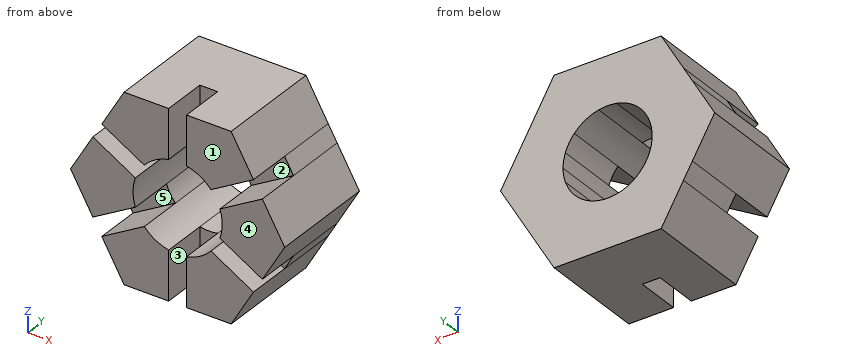
from build123d import *

# Parameters (mm, degrees)
BOSS_EXTRUDE1_DEPTH = 60
CUT_EXTRUDE1_DEPTH  = 25


with BuildPart() as part:
    # Sketch1 → Boss-Extrude1 (new body)
    with BuildSketch(Plane(origin=(0, 0, 0), x_dir=(1, 0, 0), z_dir=(0, 1, 0))):
        with BuildLine():
            Line((-47.533320997, 21.669872981), (-23.713203436, 7.917321695))
            ThreePointArc((-23.713203436, 7.917321695), (-21.650635095, 12.5), (-18.713203436, 16.577575733))
            Line((-18.713203436, 16.577575733), (-42.533320997, 30.330127019))
            Line((-42.533320997, 30.330127019), (-47.533320997, 21.669872981))
        make_face()
        with BuildLine():
            Line((-42.533320997, 30.330127019), (-18.713203436, 16.577575733))
            ThreePointArc((-18.713203436, 16.577575733), (-12.5, 21.650635095), (-5, 24.494897428))
            Line((-5, 24.494897428), (-5, 52))
            Line((-5, 52), (-30.022213998, 52))
            Line((-30.022213998, 52), (-42.533320997, 30.330127019))
        make_face()
        with BuildLine():
            Line((5, 24.494897428), (5, 52))
            Line((5, 52), (-5, 52))
            Line((-5, 52), (-5, 24.494897428))
            ThreePointArc((-5, 24.494897428), (0, 25), (5, 24.494897428))
        make_face()
        with BuildLine():
            Line((18.713203436, 16.577575733), (42.533320997, 30.330127019))
            Line((42.533320997, 30.330127019), (30.022213998, 52))
            Line((30.022213998, 52), (5, 52))
            Line((5, 52), (5, 24.494897428))
            ThreePointArc((5, 24.494897428), (12.5, 21.650635095), (18.713203436, 16.577575733))
        make_face()
        with BuildLine():
            Line((23.713203436, 7.917321695), (47.533320997, 21.669872981))
            Line((47.533320997, 21.669872981), (42.533320997, 30.330127019))
            Line((42.533320997, 30.330127019), (18.713203436, 16.577575733))
            ThreePointArc((18.713203436, 16.577575733), (21.650635095, 12.5), (23.713203436, 7.917321695))
        make_face()
        with BuildLine():
            Line((23.713203436, -7.917321695), (47.533320997, -21.669872981))
            Line((47.533320997, -21.669872981), (60.044427996, 0))
            Line((60.044427996, 0), (47.533320997, 21.669872981))
            Line((47.533320997, 21.669872981), (23.713203436, 7.917321695))
            ThreePointArc((23.713203436, 7.917321695), (24.676203982, 4.010605572), (25, 0))
            ThreePointArc((25, 0), (24.676203982, -4.010605572), (23.713203436, -7.917321695))
        make_face()
        with BuildLine():
            Line((18.713203436, -16.577575733), (42.533320997, -30.330127019))
            Line((42.533320997, -30.330127019), (47.533320997, -21.669872981))
            Line((47.533320997, -21.669872981), (23.713203436, -7.917321695))
            ThreePointArc((23.713203436, -7.917321695), (21.650635095, -12.5), (18.713203436, -16.577575733))
        make_face()
        with BuildLine():
            Line((5, -52), (30.022213998, -52))
            Line((30.022213998, -52), (42.533320997, -30.330127019))
            Line((42.533320997, -30.330127019), (18.713203436, -16.577575733))
            ThreePointArc((18.713203436, -16.577575733), (12.5, -21.650635095), (5, -24.494897428))
            Line((5, -24.494897428), (5, -52))
        make_face()
        with BuildLine():
            Line((-5, -52), (5, -52))
            Line((5, -52), (5, -24.494897428))
            ThreePointArc((5, -24.494897428), (0, -25), (-5, -24.494897428))
            Line((-5, -24.494897428), (-5, -52))
        make_face()
        with BuildLine():
            Line((-30.022213998, -52), (-5, -52))
            Line((-5, -52), (-5, -24.494897428))
            ThreePointArc((-5, -24.494897428), (-12.5, -21.650635095), (-18.713203436, -16.577575733))
            Line((-18.713203436, -16.577575733), (-42.533320997, -30.330127019))
            Line((-42.533320997, -30.330127019), (-30.022213998, -52))
        make_face()
        with BuildLine():
            Line((-47.533320997, -21.669872981), (-42.533320997, -30.330127019))
            Line((-42.533320997, -30.330127019), (-18.713203436, -16.577575733))
            ThreePointArc((-18.713203436, -16.577575733), (-21.650635095, -12.5), (-23.713203436, -7.917321695))
            Line((-23.713203436, -7.917321695), (-47.533320997, -21.669872981))
        make_face()
        with BuildLine():
            Line((-60.044427996, 0), (-47.533320997, -21.669872981))
            Line((-47.533320997, -21.669872981), (-23.713203436, -7.917321695))
            ThreePointArc((-23.713203436, -7.917321695), (-25, 0), (-23.713203436, 7.917321695))
            Line((-23.713203436, 7.917321695), (-47.533320997, 21.669872981))
            Line((-47.533320997, 21.669872981), (-60.044427996, 0))
        make_face()
    extrude(amount=BOSS_EXTRUDE1_DEPTH)

    # Sketch1_4 → Cut-Extrude1 (cut)
    with BuildSketch(Plane(origin=(0, 0, 0), x_dir=(1, 0, 0), z_dir=(0, 1, 0))):
        with BuildLine():
            Line((-47.533320997, 21.669872981), (-23.713203436, 7.917321695))
            ThreePointArc((-23.713203436, 7.917321695), (-21.650635095, 12.5), (-18.713203436, 16.577575733))
            Line((-18.713203436, 16.577575733), (-42.533320997, 30.330127019))
            Line((-42.533320997, 30.330127019), (-47.533320997, 21.669872981))
        make_face()
        with BuildLine():
            Line((-47.533320997, -21.669872981), (-42.533320997, -30.330127019))
            Line((-42.533320997, -30.330127019), (-18.713203436, -16.577575733))
            ThreePointArc((-18.713203436, -16.577575733), (-21.650635095, -12.5), (-23.713203436, -7.917321695))
            Line((-23.713203436, -7.917321695), (-47.533320997, -21.669872981))
        make_face()
        with BuildLine():
            Line((-5, -52), (5, -52))
            Line((5, -52), (5, -24.494897428))
            ThreePointArc((5, -24.494897428), (0, -25), (-5, -24.494897428))
            Line((-5, -24.494897428), (-5, -52))
        make_face()
        with BuildLine():
            Line((18.713203436, -16.577575733), (42.533320997, -30.330127019))
            Line((42.533320997, -30.330127019), (47.533320997, -21.669872981))
            Line((47.533320997, -21.669872981), (23.713203436, -7.917321695))
            ThreePointArc((23.713203436, -7.917321695), (21.650635095, -12.5), (18.713203436, -16.577575733))
        make_face()
        with BuildLine():
            Line((23.713203436, 7.917321695), (47.533320997, 21.669872981))
            Line((47.533320997, 21.669872981), (42.533320997, 30.330127019))
            Line((42.533320997, 30.330127019), (18.713203436, 16.577575733))
            ThreePointArc((18.713203436, 16.577575733), (21.650635095, 12.5), (23.713203436, 7.917321695))
        make_face()
        with BuildLine():
            Line((5, 24.494897428), (5, 52))
            Line((5, 52), (-5, 52))
            Line((-5, 52), (-5, 24.494897428))
            ThreePointArc((-5, 24.494897428), (0, 25), (5, 24.494897428))
        make_face()
    extrude(amount=CUT_EXTRUDE1_DEPTH, mode=Mode.SUBTRACT)


solid = part.part
Could you check a few things on this model? Use its own coordinates, in mm. Face numbers are marked on the shaded views. A direction names the side the tool comes from. Give positions to 0.01 mm unless a question says otherwise; leave off trailing zeros. Order: outer loops, then holes, each group sorted by start corner. A loop starts at its lowest first (then second) coordinate and runs counter-clockwise, first axis right, second up. Notation, with made-up numbers: (37.5, 87) -> (62.5, 87) arc R11 cw to (62.5, 106) -> close; hole circle Ø9 at (-34, 24.25). An arc over 180 degrees is marked (long way). Answer in a Markdown table with one row per item. Add a question column.
Item 1: For the marked faces 1, 2 and 3, which set-ups out of +Z, -Z, +X, -X, +Y, -Y let a thin tool reach every point of the face, with its end or its side?
Item 2: Imagine slicing it at B-B (x = 15). List the corners of the cut face in (y, z) for me.
Item 3: Imagine slicing it at C-C (z = -18.5). List the corners of the cut face in (x, y) for me, and give its area (3 significant figures).
Item 4: Imagine slicing it at D-D (y = 7). Count the separate pieces of the cut face and the enclosed holes in it, and give its area (3 significant figures).
Item 5: Please list where these lines run through material, in increasing order: probe 1 along Z at (x, y) = (29, 15); probe 2 along X at (y, z) = (16, 21.5); probe 3 along Z at (x, y) = (36, 17.5).
Item 6: We'd pull the mould along X, two halves only. Please class the marked faces 4 and 5: pulls with the +X half, pulls with the -X half, needs draft (parallel to the pull), parting line crosses it, or undercut.
Item 7: I'm going to push flat-ended pins straight in: P1, Ø3, axis at x = 0.5, z = 43, coming from the -Y side; P2, Ø12.5, axis at y = 15, z = -40, coming from the -X side; P3, Ø10, axis at y = 44.5, z = 19, coming from the -X side. Where does each tip first touch, or does it pass through?
Item 8: Imagine slicing it at A-A (y = 46). List the corners of the cut face in (x, z) for me.
Result:
| question | item | result |
|---|---|---|
| 1 | face 1 | +Z, -Z, +X, -X, -Y |
| 1 | face 2 | -Y |
| 1 | face 3 | +Z, -Z, -Y |
| 2 | outline | (0, -52) -> (60, -52) -> (60, -20) -> (0, -20) -> close; (0, 20) -> (60, 20) -> (60, 52) -> (0, 52) -> close |
| 3 | outline | (-49.36, 0) -> (-42.04, 0) -> (-42.04, 25) -> (-22.04, 25) -> (-22.04, 0) -> (-16.82, 0) -> (-16.82, 60) -> (-49.36, 60) -> close; (16.82, 0) -> (22.04, 0) -> (22.04, 25) -> (42.04, 25) -> (42.04, 0) -> (49.36, 0) -> (49.36, 60) -> (16.82, 60) -> close |
| 3 | area | 2,910 mm2 |
| 4 | separate pieces | 6 |
| 4 | enclosed holes | 0 |
| 4 | area | 5,770 mm2 |
| 5 | probe 1 | -52 to -22.52, -10.97 to 10.97, 22.52 to 52 |
| 5 | probe 2 | -47.63 to -47.24, -27.24 to -12.76, 12.76 to 27.24, 47.24 to 47.63 |
| 5 | probe 3 | -41.65 to -26.56, -15.01 to 15.01, 26.56 to 41.65 |
| 6 | face 4 | needs draft |
| 6 | face 5 | undercut |
| 7 | P1 | y = 25 |
| 7 | P2 | x = -40.56 |
| 7 | P3 | x = -51.96 |
| 8 | outline | (-60.04, 0) -> (-30.02, -52) -> (30.02, -52) -> (60.04, 0) -> (30.02, 52) -> (-30.02, 52) -> close; hole circle Ø50 at (0, 0) |
